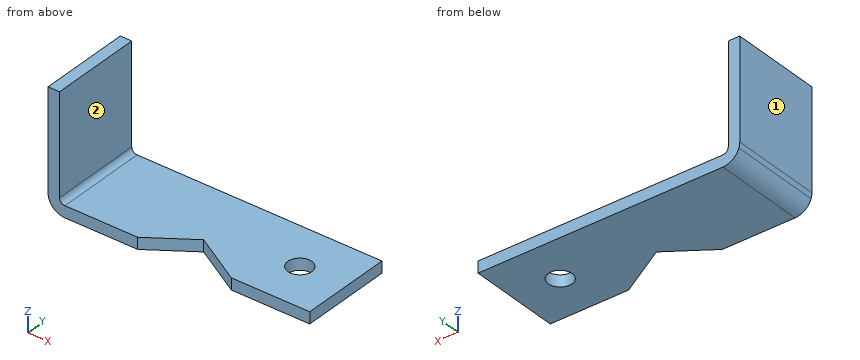
```python
from build123d import *

# Parameters (mm, degrees)
ESBO_O1_W               = 50
ESBO_O1_H               = 12.7
FLANGE_BASE1_DEPTH      = 1.5875
DOBRA_START             = -6.35
DOBRA_ESBO_ADA1_DEPTH   = 12.7
DOBRA_ESBO_ADA1_2_DEPTH = 12.7
CORTE_EXTRUS_O1_DEPTH   = 10
ESBO_O8_R               = 1.65
CORTE_EXTRUS_O2_DEPTH   = 10


# Read off the part's stored shape, not the designer's step: Dobra esboçada1
# Sheet-metal steps are written as plain solids
with BuildPart() as part:
    # Esboço1 → Flange-base1 (new body)
    with BuildSketch(Plane.XY):
        Rectangle(ESBO_O1_W, ESBO_O1_H)
    extrude(amount=-FLANGE_BASE1_DEPTH)

    # Dobra esboçada1 outline → Dobra esboçada1 (cut)
    with BuildSketch(Plane(origin=(0, 0, 0), x_dir=(1, 0, 0), z_dir=(0, 1, 0)).offset(DOBRA_START)):
        with BuildLine():
            Line((-25, 0), (-11.0023484, 0))
            ThreePointArc((-11.0023484, 0), (-10.156283273, 1.149317929), (-8.798065921, 1.5875))
            Line((-8.798065921, 1.5875), (-25, 1.5875))
            Line((-25, 1.5875), (-25, 0))
        make_face()
    extrude(amount=DOBRA_ESBO_ADA1_DEPTH, mode=Mode.SUBTRACT)

    # Dobra esbo_ada1 2 outline → Dobra esbo_ada1 2 (add)
    with BuildSketch(Plane(origin=(0, 0, 0), x_dir=(1, 0, 0), z_dir=(0, 1, 0)).offset(DOBRA_START)):
        with BuildLine():
            Line((-11.122165921, -14.534665921), (-9.534665921, -14.534665921))
            Line((-9.534665921, -14.534665921), (-9.534665921, -0.7366))
            ThreePointArc((-9.534665921, -0.7366), (-9.318920776, -0.215745145), (-8.798065921, 0))
            Line((-8.798065921, 0), (-11.0023484, 0))
            ThreePointArc((-11.0023484, 0), (-11.092015977, -0.363459343), (-11.122165921, -0.7366))
            Line((-11.122165921, -0.7366), (-11.122165921, -14.534665921))
        make_face()
    extrude(amount=DOBRA_ESBO_ADA1_2_DEPTH)

    # Esboço7 → Corte-extrusão1 (cut)
    with BuildSketch(Plane.XY):
        Polygon((1.246385816, -6.35), (7.190135396, -2.315813979), (14.178296509, -6.35), align=None)
    extrude(amount=-CORTE_EXTRUS_O1_DEPTH, mode=Mode.SUBTRACT)

    # Esboço8 → Corte-extrusão2 (cut)
    with BuildSketch(Plane.XY):
        with Locations((18.65, 0)):
            Circle(ESBO_O8_R)
    extrude(amount=-CORTE_EXTRUS_O2_DEPTH, mode=Mode.SUBTRACT)


solid = part.part
```
CAD build for the part. Positions are in the model's coordinates, mm. Face numbers are marked on the shaded views. A direction names the side the tool comes from. Coordinates: 2 decimals unless noted, no trailing zeros. Loops run counter-clockwise (first coordinate to the right, second up) from the corner with the lowest first, then second, coordinate; pieces in that order, holes last. Notation, with made-up numbers: (19, 63) - (56, 63) arc R12 ccw to (56, 84) - close; hole circle Ø7 at (10.25, 72.5). An arc over 180 degrees is marked (long way). Return JSON: item names as keys, results as strings.
1. Band-saw the part on B-B (x = 18.65). Give the cut face in (y, z), and give its area (3 significant figures).
Result:
{"outline": "(-6.35, -1.59) - (-1.65, -1.59) - (-1.65, 0) - (-6.35, 0) - close; (1.65, -1.59) - (6.35, -1.59) - (6.35, 0) - (1.65, 0) - close", "area": "14.9 mm2"}
2. Drop flat-ended pins along their axis: pin 1 (1.5 mm diameter, centred on x = 18.5, y = 3, fed in from +Z); pin 2 (3 mm diameter, centred on x = 18.65, y = 0, fed in from +Z). Give the stop position or say it passes through.
Result:
{"pin 1": "stops at z = 0", "pin 2": "passes through"}
3. Probe L1, parallel to Y at x = 18.65, z = -1; L2, parallel to X at y = -3, z = 1.25; L3, parallel to Z at x = 11, y = 5.5. List the from-to ranges inside material, lowest first. Write a range as from..to.
Result:
{"L1": "y = -6.35..-1.65, 1.65..6.35", "L2": "x = -11.12..-9.53", "L3": "z = -1.59..0"}
4. Band-saw the part on C-C (y = 4). Give the cut face in (x, z).
Result:
{"outline": "(-11.12, 0.74) arc R2.32 ccw to (-8.8, -1.59) - (25, -1.59) - (25, 0) - (-8.8, 0) arc R0.74 cw to (-9.53, 0.74) - (-9.53, 14.53) - (-11.12, 14.53) - close"}
5. Band-saw the part on D-D (z = 3). Give the cut face in (x, y).
Result:
{"outline": "(-11.12, -6.35) - (-9.53, -6.35) - (-9.53, 6.35) - (-11.12, 6.35) - close"}
6. 3-axis set-ups, long thin cutter, end or side, ignore diameter. For the marked faces 1 and 2: which of +Z, -Z, +X, -X, +Y, -Y reach the whole face in a straight line?
Result:
{"face 1": "+Z, -Z, -X, +Y, -Y", "face 2": "+Z, +X, +Y, -Y"}
7. Band-saw the part on A-A (y = 0). Give the cut face in (x, z).
Result:
{"outline": "(-11.12, 0.74) arc R2.32 ccw to (-8.8, -1.59) - (17, -1.59) - (17, 0) - (-8.8, 0) arc R0.74 cw to (-9.53, 0.74) - (-9.53, 14.53) - (-11.12, 14.53) - close; (20.3, -1.59) - (25, -1.59) - (25, 0) - (20.3, 0) - close"}
